The model under review builds one solid part; all positions refer to its coordinate system, in mm. A direction names the side the tool comes from. Coordinates: 2 decimals unless noted, no trailing zeros. Loops run counter-clockwise (first coordinate to the right, second up) from the corner with the lowest first, then second, coordinate; pieces in that order, holes last. Notation, with made-up numbers: (64.5, 14) - (123.5, 14) arc R10 ccw to (123.5, 18) - close; hole circle Ø9 at (-9, -16). An arc over 180 degrees is marked (long way). Answer in a Markdown table with one row per item. Add a question column.
(1) For P1, Ø2.5, axis at x = 12.4, z = 0, coming from the +Y side; P2, Ø5.5, axis at x = -12.4, z = 0, coming from the +Y side, all flat-tipped, find the tip position at first contact; note any pin that passes through.
(2) We need section A-A on x = 0. Write out the cut boundary in (y, z).
(3) We need section B-B on z = 0. Give the number of separate pieces and of enclosed holes in the cut face, plus the area to 3 significant figures.
(4) For line 1 along X through (y, z) = (-4.35, 0); line 2 along Y through (x, z) = (19.4, 0); line 3 along Z through (x, y) = (-12.4, 4.2), list the stretches that pass through material, from the lowest coordinate up.
(5) Mouldability with a two-part tool opening along Z and no side actions: class faces 3 (the flat face through (-20, -0.1, 3.4)), 4 (the cylindrical face through (-10.397, 5.146, -0.631)), 5 (the flat face through (0, -4, -7.8)) as +Z half, -Z half, draft (parallel to the pull), parting line (faces both ways), or undercut.
(6) We need section D-D on x = 15.5. Write out the cut boundary in (y, z).
(7) Machinability: for faces 1 (the cylindrical face through (14.34, 5.15, 0.8)), 2 (the cylindrical face through (18.669, 1.262, -4.006)), which of the approach directions +Z, -Z, +X, -X, +Y, -Y give a long, thin tool a straight path to every point of the face, cutting with its end or side? Answer none if there is none.
(8) We need section C-C on y = 0. Write out the cut boundary in (x, z).
Autodesk Inventor part; units mm, degrees
sketch "Эскиз1" plane through (0, 0, 0) normal (0, 1, 0) x (-1, 0, 0)
  line L0 (20, 7.8) -> (-20, 7.8)
  line L1 (-20, 7.8) -> (-20, -7.8)
  line L2 (-20, -7.8) -> (20, -7.8)
  line L3 (20, -7.8) -> (20, 7.8)
  line L4 (20, 7.8) -> (-20, -7.8) construction
  line L5 (-20, 7.8) -> (20, -7.8) construction
  point P0 (0, 0)
  dimension "d0" = 40
  dimension "d1" = 15.6
extrude "Выдавливание1" add sketch "Эскиз1" along normal mid plane 16
sketch "Эскиз2" plane through (20, -8, -7.8) normal (1, 0, 0) x (0, 0, -1)
  circle A0 centre (-7.8, 8) radius 3.05
  dimension "d4" = 6.1
extrude "Выдавливание2" cut sketch "Эскиз2" against normal up to next
sketch "Эскиз3" plane through (0, 8, 0) normal (0, 1, 0) x (1, 0, 0)
  circle A0 centre (-12.4, 0) radius 2.1
  circle A1 centre (12.4, 0) radius 2.1
  line L0 (28, 0) -> (-28, 0)
  line L1 (0, 10.92) -> (0, -10.92)
  line L2 (-20, 7.8) -> (-20, -7.8)
  line L3 (20, -7.8) -> (20, 7.8)
  point P0 (0, 0)
  dimension "d7" = 4.2
  dimension "d9" = 7.6
  dimension "d10" = 7.6
extrude "Выдавливание3" cut sketch "Эскиз3" against normal blind 21.75
sketch "Эскиз4" plane through (-20, 8, 7.8) normal (0, 0, 1) x (1, 0, 0)
  circle A0 centre (20, -8) radius 2.1
  dimension "d13" = 4.2
extrude "Выдавливание4" cut sketch "Эскиз4" against normal blind 19.55
sketch "Эскиз5" plane through (20, -8, -7.8) normal (1, 0, 0) x (0, 0, -1)
  circle A0 centre (-7.8, 8) radius 3.5
  circle A1 centre (-7.8, 8) radius 3.05
  dimension "d17" = 7
extrude "Выдавливание5" add sketch "Эскиз5" along normal blind 5.3
sketch "Эскиз6" plane through (20, -8, -7.8) normal (1, 0, 0) x (0, 0, -1)
  circle A0 centre (-7.8, 8) radius 3.5
  circle A1 centre (-7.8, 8) radius 4.2
  dimension "d20" = 8.4
extrude "Выдавливание6" cut sketch "Эскиз6" against normal blind 2.7
properties part number "новое крепление штыря стрелялки"
Outcome:
| question | item | result |
|---|---|---|
| 1 | P1 | through |
| 1 | P2 | y = 8 |
| 2 | outline | (-8, -7.8) - (-2.1, -7.8) - (-2.1, -2.21) arc R3.05 cw to (-2.1, 2.21) - (-2.1, 7.8) - (-8, 7.8) - close; (2.1, -7.8) - (8, -7.8) - (8, 7.8) - (2.1, 7.8) - (2.1, 2.21) arc R3.05 cw to (2.1, -2.21) - close |
| 3 | separate pieces | 6 |
| 3 | enclosed holes | 0 |
| 3 | area | 314 mm² |
| 4 | line 1 | -20 to -14.5, -10.3 to 10.3, 14.5 to 20 |
| 4 | line 2 | -8 to -4.2, -3.5 to -3.05, 3.05 to 3.5, 4.2 to 8 |
| 4 | line 3 | -7.8 to -2.1, 2.1 to 7.8 |
| 5 | face 3 | draft |
| 5 | face 4 | undercut |
| 5 | face 5 | -Z half |
| 6 | outline | (-8, -7.8) - (8, -7.8) - (8, 7.8) - (-8, 7.8) - close; hole circle Ø6.1 at (0, 0) |
| 7 | face 1 | +Y, -Y |
| 7 | face 2 | +X |
| 8 | outline | (-20, -7.8) - (-2.1, -7.8) - (-2.1, -3.05) - (-20, -3.05) - close; (-20, 3.05) - (-2.1, 3.05) - (-2.1, 7.8) - (-20, 7.8) - close; (2.1, -7.8) - (20, -7.8) - (20, -4.2) - (17.3, -4.2) - (17.3, -3.5) - (25.3, -3.5) - (25.3, -3.05) - (2.1, -3.05) - close; (2.1, 3.05) - (25.3, 3.05) - (25.3, 3.5) - (17.3, 3.5) - (17.3, 4.2) - (20, 4.2) - (20, 7.8) - (2.1, 7.8) - close |
